```python
from build123d import *

# Parameters (mm, degrees)
F0_W      = 90
F0_H      = 45
F1_DEPTH  = 25
F3_DEPTH  = 8
F6_DEPTH  = 8
F8_DEPTH  = 8
F11_DEPTH = 8
F13_DEPTH = 100


with BuildPart() as f1:
    # F0 (on Front) → F1 (new body)
    with BuildSketch(Plane.XZ):
        with Locations((-17.625819491, 22.5)):
            Rectangle(F0_W, F0_H)
    extrude(amount=F1_DEPTH)

    # F2 (on face) → F3 (join)
    with BuildSketch(Plane(origin=(-62.625819491, 0, 0), x_dir=(0, -1, 0), z_dir=(-1, 0, 0))):
        Polygon((8.3801829397, 0), (6.88952161, 0), (6.88952161, -6.5082041547), (10.5835897848, -10.7495421544), (17.287639901, -10.7495421544), (18.5189954937, -9.3129593879), (16.0562843084, -9.3129593879), (15.1669709012, -9.9286381155), (11.2676769495, -9.9286381155), (8.3801829397, -6.6133668514), align=None)
    extrude(amount=-F3_DEPTH)

    # F5 (on offset) → F6 (join)
    with BuildSketch(Plane(origin=(-37.625819491, 0, 0), x_dir=(0, -1, 0), z_dir=(-1, 0, 0))):
        Polygon((8.3582568914, 0), (6.8190610036, 0), (6.8190610036, -6.4087822102), (10.5131296441, -10.6843244284), (17.3197928816, -10.6843244284), (18.5169447213, -9.3503547832), (16.0542316735, -9.3503547832), (15.233328566, -9.931829758), (11.2656243145, -9.931829758), (8.3582568914, -6.5456000157), align=None)
    extrude(amount=-F6_DEPTH)

    # F7 (on face) → F8 (join)
    with BuildSketch(Plane.YZ.offset(27.374180509)):
        Polygon((-6.7952279933, 0), (-8.3815939724, 0), (-8.3409175277, -6.5609556623), (-11.2289162353, -9.7336871549), (-15.0931403041, -9.7336871549), (-15.9473381937, -9.2862509191), (-18.3878988028, -9.2862509191), (-17.208294943, -10.5878841132), (-10.4560721666, -10.5878841132), (-6.7952279933, -6.438927725), align=None)
    extrude(amount=-F8_DEPTH)

    # F10 (on offset) → F11 (join)
    with BuildSketch(Plane.YZ.offset(2.374180509)):
        Polygon((-6.8191965111, 0), (-8.4298858419, 0), (-8.3435988054, -6.4949798398), (-11.248591356, -9.946456179), (-15.3903635219, -9.946456179), (-16.0806588829, -9.2849237844), (-18.4966921806, -9.2849237844), (-17.1736273915, -10.63675154), (-10.558295995, -10.63675154), (-6.8191965111, -6.4662178047), align=None)
    extrude(amount=-F11_DEPTH)

    # F12 (on face) → F13 (cut)
    with BuildSketch(Plane.YZ.offset(27.374180509)):
        Polygon((-14.3797518685, -0.9674453177), (-14.3797518685, 0), (-14.3797518685, 45.9536239505), (-25.8923433721, 45.9536239505), (-25.8923433721, -0.9674453177), align=None)
    extrude(amount=-F13_DEPTH, mode=Mode.SUBTRACT)


solid = f1.part
```
Work out the finished part from the listing and answer in its coordinate system (mm). A direction names the side the tool comes from. Give positions to 0.01 mm unless a question says otherwise; leave off trailing zeros. Loops run counter-clockwise (first coordinate to the right, second up) from the corner with the lowest first, then second, coordinate; pieces in that order, holes last. Notation, with made-up numbers: (22.5, 15.25) -> (48.5, 15.25) arc R15 cw to (48.5, 25.25) -> close; hole circle Ø2 at (58.5, -9). An arc over 180 degrees is marked (long way). Write item = value, one per line. Start each with the question number.
(1) Given pin 1 Ø7.5 at (x, z) = (-58, -3) entering from -Y; pin 2 Ø1.9 at (x, z) = (25, -2) entering from +Y; pin 3 Ø8.5 at (y, z) = (-13.5, -4) entering from -X; pin 4 Ø2.5 at (x, y) = (-34.5, -17) entering from +Z, each flat-ended and moving along its own axis, determine where each tip first touches the part or whether it passes through.
(2) Find section C-C on z = 38. Give the vertices of the cut face in (x, y).
(3) Which of the six approach directions +Z, -Z, +X, -X, +Y, -Y give full straight-line access (tool end or side, diameter ignored) to faces 4 (the flat face through (-59, -13, -9.929)), 5 (the flat face through (23, -6.795, -3)), 6 (the flat face through (-2, -17, -9.285)), 7 (the flat face through (-34, -14, -10.684))?
(4) Find the intervals of material crossed by probe 1 along X at (y, z) = (-7, -5.5); probe 2 along Z at (x, y) = (-5.5, -11.5); probe 3 along Y at (x, z) = (-29, 12.5), in increasing order. Write a range as from..to.
(5) Find section B-B on x = -6.5. Give the vertices of the cut face in (y, z).
(6) Find section A-A on y = -13.25. Give the vertices of the cut face in (x, z).
(7) The mould has two halves that part along X. Classify faces 1 (the flat face through (19.374, -8, -6)), 2 (the flat face through (2.374, -8.8, -7.3)), 3 (the flat face through (-62.626, -7, 23)): +X half, -X half, draft (parallel to the pull), parting line (faces both ways), or undercut.
From the geometry:
q1.pin_1 = -14.38
q1.pin_2 = -6.8
q1.pin_3 = -62.63
q1.pin_4 = -9.35
q2.outline = (-62.63, -14.38) -> (27.37, -14.38) -> (27.37, 0) -> (-62.63, 0) -> close
q3.face_4 = -X
q3.face_5 = -Z, +X, -X, +Y
q3.face_6 = +Z, +X, -X, -Y
q3.face_7 = -Z, +X, +Y, -Y
q4.probe_1 = -62.63..-54.63, -37.63..-29.63, -5.63..2.37, 19.37..27.37
q4.probe_2 = -10.64..-9.95, 0..45
q4.probe_3 = -14.38..0
q5.outline = (-14.38, 0) -> (0, 0) -> (0, 45) -> (-14.38, 45) -> close
q6.outline = (-62.63, -10.75) -> (-54.63, -10.75) -> (-54.63, -9.93) -> (-62.63, -9.93) -> close; (-62.63, 0) -> (27.37, 0) -> (27.37, 45) -> (-62.63, 45) -> close; (-37.63, -10.68) -> (-29.63, -10.68) -> (-29.63, -9.93) -> (-37.63, -9.93) -> close; (-5.63, -10.64) -> (2.37, -10.64) -> (2.37, -9.95) -> (-5.63, -9.95) -> close; (19.37, -10.59) -> (27.37, -10.59) -> (27.37, -9.73) -> (19.37, -9.73) -> close
q7.face_1 = undercut
q7.face_2 = undercut
q7.face_3 = -X half
